from build123d import *

# Parameters (mm, degrees)
SKETCH1_R           = 2.127
SKETCH1_R_2         = 2.032
BOSS_EXTRUDE1_DEPTH = 44.958
SKETCH2_W           = 61.162711876
SKETCH2_H           = 56.657422832
CUT_EXTRUDE1_DEPTH  = 57.200072865


with BuildPart() as part:
    # Sketch1 → Boss-Extrude1 (new body)
    with BuildSketch(Plane.XY):
        with BuildLine():
            Line((6.662551774, -21.675328207), (9.781210426, 28.223210221))
            ThreePointArc((9.781210426, 28.223210221), (8.75546188, 31.069569496), (5.978630102, 32.270871491))
            Line((5.978630102, 32.270871491), (-5.353526553, 32.270871491))
            ThreePointArc((-5.353526553, 32.270871491), (-8.130358331, 31.069569496), (-9.156106877, 28.223210221))
            Line((-9.156106877, 28.223210221), (-6.037448226, -21.675328207))
            ThreePointArc((-6.037448226, -21.675328207), (0.312551774, -27.895146648), (6.662551774, -21.675328207))
        make_face()
        with Locations((0.312551774, -22.815146648)):
            Circle(SKETCH1_R, mode=Mode.SUBTRACT)
        with Locations((0.312551774, 0.044853352)):
            Circle(SKETCH1_R, mode=Mode.SUBTRACT)
        with Locations((0.312551774, 22.110871491)):
            Circle(SKETCH1_R_2, mode=Mode.SUBTRACT)
    extrude(amount=BOSS_EXTRUDE1_DEPTH)

    # Sketch2 → Cut-Extrude1 (cut, through all)
    with BuildSketch(Plane.XY.offset(44.958)):
        with Locations((2.830749484, 9.323564768)):
            Rectangle(SKETCH2_W, SKETCH2_H)
    extrude(amount=-CUT_EXTRUDE1_DEPTH, mode=Mode.SUBTRACT)


solid = part.part
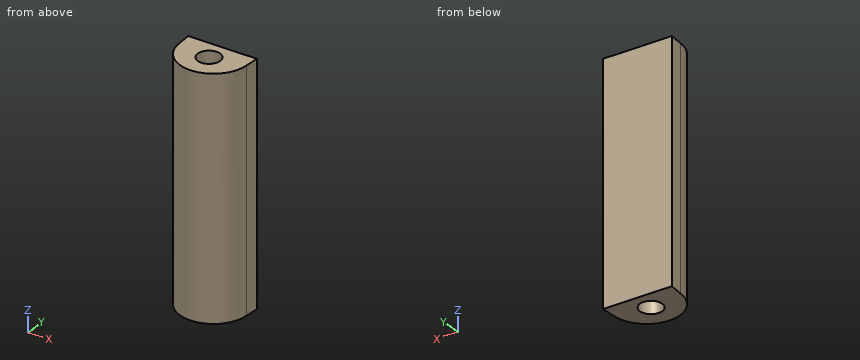
For this review, take the finished solid that the model builds, in its own axes (mm). Give positions to 0.01 mm unless a question says otherwise; leave off trailing zeros. Order: outer loops, then holes, each group sorted by start corner. A loop starts at its lowest first (then second) coordinate and runs counter-clockwise, first axis right, second up. Notation, with made-up numbers: (-19, 30.25) -> (16, 30.25) arc R27 ccw to (16, 51.25) -> close; hole circle Ø7 at (4, 80.25). An arc over 180 degrees is marked (long way). Write item = value, one per line.
1) We need section D-D, the plane x = 5.25. Give the boundary of the cut face in (y, z), and give its area (3 significant figures).
Findings:
outline = (-25.54, 0) -> (-19.01, 0) -> (-19.01, 44.96) -> (-25.54, 44.96) -> close
area = 294 mm^2
2) To check wall thickness, follow L1, parallel to Y at x = 0.5, z = 12; L2, parallel to X at y = -23.5, z = 25; L3, parallel to Y at x = -1.5, z = 32.5. State the ranges of each line that lie inside material, in increasing order. Write a range as from..to.
Findings:
L1 = -27.89..-24.93, -20.7..-19.01
L2 = -5.73..-1.7, 2.33..6.36
L3 = -27.63..-23.93, -21.7..-19.01
3) Insertion check: pin 1 (2 mm diameter, centred on y = -26.5, z = 29, fed in from +X); pin 2 (3 mm diameter, centred on y = -25.5, z = 29.5, fed in from -X); pin 3 (3.5 mm diameter, centred on x = 0.31, y = -22.82, fed in from -Z); pin 4 (3 mm diameter, centred on y = -26.5, z = 17.5, fed in from +X). Each pin has a flat end and moves straight along its axis. Give the tip position at first contact, or say it passes through.
Findings:
pin_1 = 5.28
pin_2 = -5.54
pin_3 = through
pin_4 = 5.64
4) We need section B-B, the plane x = -1.25. Give the boundary of the cut face in (y, z), and give its area (3 significant figures).
Findings:
outline = (-27.7, 0) -> (-24.26, 0) -> (-24.26, 44.96) -> (-27.7, 44.96) -> close; (-21.37, 0) -> (-19.01, 0) -> (-19.01, 44.96) -> (-21.37, 44.96) -> close
area = 261 mm^2
5) We need section A-A, the plane y = -22.25. Give the boundary of the cut face in (x, z), and give its area (3 significant figures).
Findings:
outline = (-6, 0) -> (-1.74, 0) -> (-1.74, 44.96) -> (-6, 44.96) -> close; (2.36, 0) -> (6.62, 0) -> (6.62, 44.96) -> (2.36, 44.96) -> close
area = 383 mm^2
